```python
from build123d import *

# Parameters (mm, degrees)
F1_DEPTH = 20
F2_R     = 1.5
F3_R     = 3.5
F4_R     = 2


with BuildPart() as f1:
    # F0 (on Top) → F1 (new body)
    with BuildSketch(Plane.XY):
        with BuildLine():
            Line((0, 1.2), (0, 0))
            Line((0, 0), (40, 0))
            Line((40, 0), (40, 0.334315))
            Line((40, 0.334315), (40, 1.465685))
            Line((40, 1.465685), (40, 2.834315))
            Line((40, 2.834315), (40, 3.965685))
            Line((40, 3.965685), (40, 5.334315))
            Line((40, 5.334315), (40, 6.465685))
            Line((40, 6.465685), (40, 7.834315))
            Line((40, 7.834315), (40, 8.965685))
            Line((40, 8.965685), (40, 12))
            Line((40, 12), (46, 12))
            Line((46, 12), (46, 8.965685))
            Line((46, 8.965685), (46, 7.834315))
            Line((46, 7.834315), (46, 6.465685))
            Line((46, 6.465685), (46, 5.334315))
            Line((46, 5.334315), (46, 3.965685))
            Line((46, 3.965685), (46, 2.834315))
            Line((46, 2.834315), (46, 1.465685))
            Line((46, 1.465685), (46, 0.334315))
            Line((46, 0.334315), (46, 0))
            Line((46, 0), (48, 0))
            Line((48, 0), (48, 14))
            Line((48, 14), (38, 14))
            Line((38, 14), (38, 1.2))
            Line((38, 1.2), (4, 1.2))
            ThreePointArc((4, 1.2), (2, 3.2), (0, 1.2))
        make_face()
        Polygon((40, 1.465685), (40, 0.334315), (42.6, 2.934315), (42.034315, 3.5), align=None)
        Polygon((40, 3.965685), (40, 2.834315), (42.6, 5.434315), (42.034315, 6), align=None)
        Polygon((40, 6.465685), (40, 5.334315), (42.6, 7.934315), (42.034315, 8.5), align=None)
        Polygon((40, 8.965685), (40, 7.834315), (42.6, 10.434315), (42.034315, 11), align=None)
        Polygon((46, 7.834315), (46, 8.965685), (43.965685, 11), (43.4, 10.434315), align=None)
        Polygon((43.4, 7.934315), (46, 5.334315), (46, 6.465685), (43.965685, 8.5), align=None)
        Polygon((43.4, 5.434315), (46, 2.834315), (46, 3.965685), (43.965685, 6), align=None)
        Polygon((43.4, 2.934315), (46, 0.334315), (46, 1.465685), (43.965685, 3.5), align=None)
    extrude(amount=F1_DEPTH)

    # F2
    f2_edges = [f1.edges().sort_by_distance(p)[0] for p in [
        (40, 12, 10),
        (46, 12, 10),
    ]]
    fillet(f2_edges, radius=F2_R)

    # F3
    f3_edges = [f1.edges().sort_by_distance(p)[0] for p in [
        (38, 14, 10),
        (48, 14, 10),
    ]]
    fillet(f3_edges, radius=F3_R)

    # F4
    f4_edges = [f1.edges().sort_by_distance(p)[0] for p in [
        (38, 1.2, 10),
    ]]
    fillet(f4_edges, radius=F4_R)


solid = f1.part
```
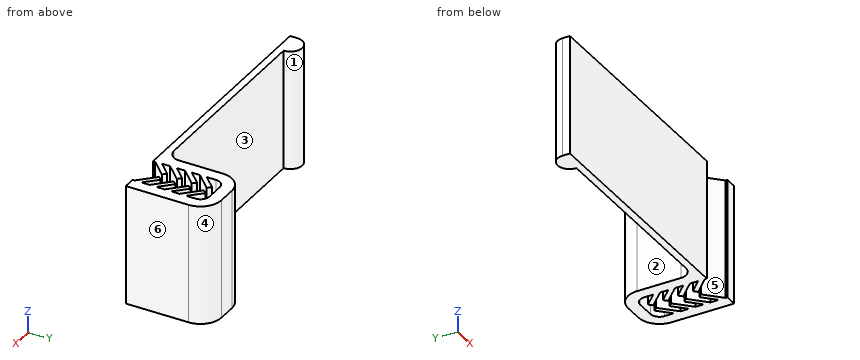
The listing builds one solid part. Answer for the finished solid, in the listing's coordinates (mm). Face numbers are marked on the shaded views. A direction names the side the tool comes from. Coordinates: 2 decimals unless noted, no trailing zeros. Write each loop counter-clockwise with the first axis right and the second up, starting at its lowest first coordinate (ties: lowest second). Pieces come first, ordered by that corner, then holes. Notation, with made-up numbers: (33.5, 83.5) - (37.5, 83.5) arc R18 ccw to (37.5, 106.5) - close; hole circle Ø1 at (-36, 89.25). An arc over 180 degrees is marked (long way). One line per item, written item: value.
1) For a pull along X with two mould halves and no side action, classify the marked faces 1, 2, 3 and 4 as pulls with the +X half, pulls with the -X half, needs draft (parallel to the pull), parting line crosses it, or undercut.
Geometry check:
face 1: undercut
face 2: pulls with the -X half
face 3: undercut
face 4: pulls with the +X half
2) Find section A-A (y = 11.5). Give the vertices of the cut face in (x, z), and give its area (3 significant figures).
Geometry check:
outline: (38.15, 0) - (40.38, 0) - (40.38, 20) - (38.15, 20) - close; (45.62, 0) - (47.85, 0) - (47.85, 20) - (45.62, 20) - close
area: 89.4 mm2
3) Find section C-C (x = 32). Give the vertices of the cut face in (y, z).
Geometry check:
outline: (0, 0) - (1.2, 0) - (1.2, 20) - (0, 20) - close
4) A tool of negligible diameter and unlimited length cuts with its end or side. For the marked faces 5 and 6, from which of +Z, -Z, +X, -X, +Y, -Y can it reach the whole face along a straight path? Write none if from no direction.
Geometry check:
face 5: +Z, -Z, -Y
face 6: +Z, -Z, +X, +Y, -Y
5) Find section B-B (x = 2). Give the vertices of the cut face in (y, z).
Geometry check:
outline: (0, 0) - (3.2, 0) - (3.2, 20) - (0, 20) - close
6) Each of these flat-tipped pins is pushed along its axis until it touches: pin 1 Ø3 at (x, z) = (32.5, 5.5) entering from +Y; pin 2 Ø12 at (x, z) = (34, 3.5) entering from +Y; pin 3 Ø0.7 at (y, z) = (2.5, 10) entering from -X. Where does it stop, or does it pass through?
Geometry check:
pin 1: stops at y = 1.2
pin 2: stops at y = 13.66
pin 3: stops at x = 0.24
7) Consider line 1 along X through (y, z) = (3, 8); line 2 along X through (y, z) = (7, 17.25); line 3 along X through (y, z) = (10.75, 14.5). Determine where each line is inside the solid, lowest interval first. Write a range as from..to.
Geometry check:
line 1: x = 1.13..2.87, 37.99..40.17, 41.53..42.53, 43.47..44.47, 45.83..48
line 2: x = 38..40, 40.53..41.67, 44.33..45.47, 46..48
line 3: x = 38.01..40.02, 41.78..42.28, 43.72..44.22, 45.98..47.99
